```python
from build123d import *

# Parameters (mm, degrees)
SKETCH2_R           = 6.25
BOSS_EXTRUDE1_DEPTH = 14
SKETCH4_R           = 1.75
CUT_EXTRUDE1_DEPTH  = 5.5
CUT_EXTRUDE2_START  = -14
SKETCH4_3_R         = 3.375
CUT_EXTRUDE2_DEPTH  = 5.5


with BuildPart() as part:
    # Sketch2 → Boss-Extrude1 (new body)
    with BuildSketch(Plane.XY):
        Circle(SKETCH2_R)
    extrude(amount=BOSS_EXTRUDE1_DEPTH)

    # Sketch4 → Cut-Extrude1 (cut)
    with BuildSketch(Plane.XY.offset(14)):
        Circle(SKETCH4_R)
    extrude(amount=-CUT_EXTRUDE1_DEPTH, mode=Mode.SUBTRACT)

    # Sketch4<3> → Cut-Extrude2 (cut)
    with BuildSketch(Plane.XY.offset(14).offset(CUT_EXTRUDE2_START)):
        Circle(SKETCH4_3_R)
    extrude(amount=CUT_EXTRUDE2_DEPTH, mode=Mode.SUBTRACT)


solid = part.part
```
Can you work these out from the model? Positions are in its coordinate system, mm. A direction names the side the tool comes from. Give positions to 0.01 mm unless a question says otherwise; leave off trailing zeros. Order: outer loops, then holes, each group sorted by start corner. A loop starts at its lowest first (then second) coordinate and runs counter-clockwise, first axis right, second up. Notation, with made-up numbers: M 67.5,68.5 L 103.5,68.5 A15 ccw 103.5,72.5 Z; hole C -32,2.25 d7. An arc over 180 degrees is marked long. Write item = value, one per line. Start each with the question number.
Q1. For faces 4 (the flat face through (3, -3, 0)), 5 (the flat face through (0, 0, 5.5)), 6 (the flat face through (0, 0, 8.5)), which set-ups out of +Z, -Z, +X, -X, +Y, -Y let a thin tool reach every point of the face, with its end or its side?
Q2. I need wall thicknesses on probe 1 along Y at (x, z) = (0, 1.75) (3 decimals); probe 2 along Y at (x, z) = (0, 12.05); probe 3 along X at (y, z) = (2, 3.5). Which ranges of each line are inside material? Lowest first, please. Write a range as [from, to].
Q3. Suppose I cut it at A-A (x = 0). Write out the boundary of the cut face in (y, z) (3 decimals).
Q4. We'd pull the mould along Y, two halves only. Please class faces 1 (the cylindrical face through (1.617, -0.67, 11.288)), 2 (the flat face through (-1.5, -1.3, 14)), 3 (the cylindrical face through (5.96, 1.88, 6.9)): pulls with the +Y half, pulls with the -Y half, needs draft (parallel to the pull), parting line crosses it, or undercut.
Q5. Suppose I cut it at D-D (z = 7). Write out the boundary of the cut face in (x, y), plus the area to 3 significant figures.
Q6. Suppose I cut it at C-C (z = 4.5). Write out the boundary of the cut face in (x, y) (3 decimals).
Q7. Will these pins go through, and if not, where does the flat tip stop? pin 1 Ø3 at (x, z) = (-4, 5) entering from -Y; pin 2 Ø2 at (x, y) = (0, 0) entering from -Z; pin 3 Ø5 at (x, z) = (3.5, 4.5) entering from -Y.
Check result:
q1.face_4 = -Z, +X, -X, +Y, -Y
q1.face_5 = -Z
q1.face_6 = +Z
q2.probe_1 = [-6.25, -3.375], [3.375, 6.25]
q2.probe_2 = [-6.25, -1.75], [1.75, 6.25]
q2.probe_3 = [-5.92, -2.72], [2.72, 5.92]
q3.outline = M -6.25,0 L -3.375,0 L -3.375,5.5 L 3.375,5.5 L 3.375,0 L 6.25,0 L 6.25,14 L 1.75,14 L 1.75,8.5 L -1.75,8.5 L -1.75,14 L -6.25,14 Z
q4.face_1 = undercut
q4.face_2 = needs draft
q4.face_3 = parting line crosses it
q5.outline = C 0,0 d12.5
q5.area = 123 mm2
q6.outline = C 0,0 d12.5; hole C 0,0 d6.75
q7.pin_1 = -5.73
q7.pin_2 = 5.5
q7.pin_3 = -6.17
